from build123d import *

# Parameters (mm, degrees)
F1_DEPTH = 31.75


with BuildPart() as f1:
    # F0 (on Front) → F1 (new body)
    with BuildSketch(Plane.XZ):
        with BuildLine():
            Line((-39.437188, 62.446829), (-39.916299, 62.446829))
            Line((-39.916299, 62.446829), (-39.916299, -62.446829))
            Line((-39.916299, -62.446829), (39.916299, -62.446829))
            Line((39.916299, -62.446829), (39.916299, 62.446829))
            Line((39.916299, 62.446829), (39.437188, 62.446829))
            ThreePointArc((39.437188, 62.446829), (0, 101.884017), (-39.437188, 62.446829))
        make_face()
        with BuildLine():
            ThreePointArc((-18.085412, 62.446829), (0, 80.532241), (18.085412, 62.446829))
            ThreePointArc((18.085412, 62.446829), (0, 44.361417), (-18.085412, 62.446829))
        make_face(mode=Mode.SUBTRACT)
    extrude(amount=F1_DEPTH)


solid = f1.part
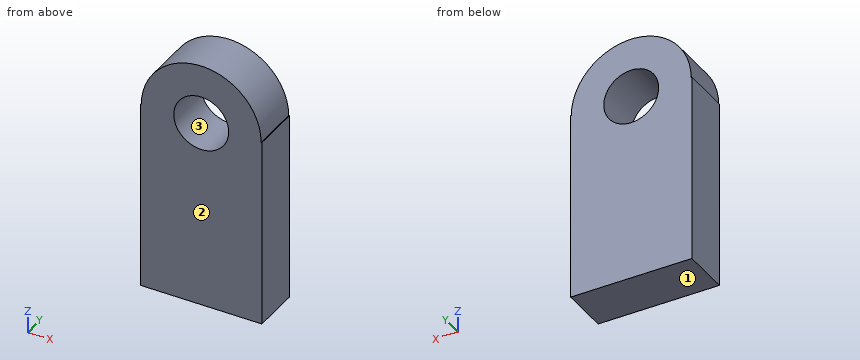
Build history of the part. All positions in model axes, mm. Face numbers are marked on the shaded views. Round coordinates to 2 decimals unless told otherwise and drop trailing zeros. Write each loop counter-clockwise with the first axis right and the second up, starting at its lowest first coordinate (ties: lowest second). Pieces come first, ordered by that corner, then holes. Notation, with made-up numbers: M 74,33.5 L 93,33.5 A28 ccw 93,65.5 Z; hole C 57,64 d4. An arc over 180 degrees is marked long. Use CSV: the item, a comma, the result in double quotes.
1. Saw through at A-A (x = 0). Give the cut face in (y, z), plus the area to 3 significant figures.
Reply:
outline,"M -31.75,-62.45 L 0,-62.45 L 0,44.36 L -31.75,44.36 Z; M -31.75,80.53 L 0,80.53 L 0,101.88 L -31.75,101.88 Z"
area,"4,070 mm²"
2. Two-plate mould, pull along Z, no slides. Class the marked faces 1, 2 and 3: +Z half, -Z half, draft (parallel to the pull), parting line (faces both ways), or undercut.
Reply:
face 1,"-Z half"
face 2,"draft"
face 3,"undercut"
3. Saw through at D-D (x = 27). Give the cut face in (y, z).
Reply:
outline,"M -31.75,-62.45 L 0,-62.45 L 0,91.19 L -31.75,91.19 Z"
4. Wall check: probe 1 along Z at (x, y) = (0, -12); probe 2 along X at (y, z) = (-8, 62.5); probe 3 along Z at (x, y) = (-6, -25). Give the ranges that are in metal, low to high. Write a range as from..to.
Reply:
probe 1,"z = -62.45..44.36, 80.53..101.88"
probe 2,"x = -39.44..-18.09, 18.09..39.44"
probe 3,"z = -62.45..45.39, 79.51..101.42"
5. Flat gauge pins, fed straight in: pin 1 (10 mm diameter, centred on x = -32, z = 24.5, fed in from +Y); pin 2 (1.5 mm diameter, centred on y = -25.5, z = 74, fed in from -X); pin 3 (8 mm diameter, centred on x = -8, z = 53.5, fed in from +Y); pin 4 (12 mm diameter, centred on x = -18, y = -22, fed in from +Z). Where does each tip first touch, or does it go through?
Reply:
pin 1,"stops at y = 0"
pin 2,"stops at x = -37.93"
pin 3,"passes through"
pin 4,"stops at z = 100.01"
6. Saw through at B-B (y = -3). Give the cut face in (x, z).
Reply:
outline,"M -39.92,-62.45 L 39.92,-62.45 L 39.92,62.45 L 39.44,62.45 A39.44 ccw -39.44,62.45 L -39.92,62.45 Z; hole C 0,62.45 d36.17"
7. Saw through at C-C (z = 48.5). Give the cut face in (x, y), plus the area to 3 significant figures.
Reply:
outline,"M -39.92,-31.75 L -11.51,-31.75 L -11.51,0 L -39.92,0 Z; M 11.51,-31.75 L 39.92,-31.75 L 39.92,0 L 11.51,0 Z"
area,"1,800 mm²"
